from build123d import *

# Parameters (mm, degrees)
F0_W     = 4
F0_H     = 3.5
F1_DEPTH = 0.3


with BuildPart() as f1:
    # F0 (on Right) → F1 (new body)
    with BuildSketch(Plane.YZ):
        Polygon((-75.175237, 25.629358), (-80.175237, 25.629358), (-80.175237, 21.129358), (-80.175237, 20.129358), (-80.175237, 15.629358), (-75.175237, 15.629358), (-74.175237, 15.629358), (-69.175237, 15.629358), (-69.175237, 20.129358), (-69.175237, 21.129358), (-69.175237, 25.629358), (-74.175237, 25.629358), align=None)
        with Locations((-77.175237, 18.379358)):
            Rectangle(F0_W, F0_H, mode=Mode.SUBTRACT)
        with Locations((-72.175237, 18.379358)):
            Rectangle(F0_W, F0_H, mode=Mode.SUBTRACT)
        with Locations((-77.175237, 22.879358)):
            Rectangle(F0_W, F0_H, mode=Mode.SUBTRACT)
        with Locations((-72.175237, 22.879358)):
            Rectangle(F0_W, F0_H, mode=Mode.SUBTRACT)
    extrude(amount=F1_DEPTH)


solid = f1.part
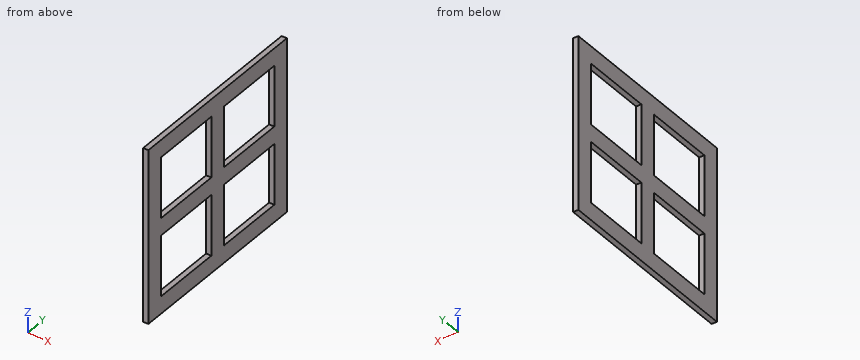
Can you work these out from the model? Positions are in its coordinate system, mm. Coordinates: 2 decimals unless noted, no trailing zeros. Loops run counter-clockwise (first coordinate to the right, second up) from the corner with the lowest first, then second, coordinate; pieces in that order, holes last. Notation, with made-up numbers: M 53.5,53 L 64.5,53 A30 ccw 64.5,80 Z; hole C -21.75,71 d4. An arc over 180 degrees is marked long. Answer as CSV lines item,"result". Start each with the question number.
1. Suppose I cut it at B-B, the plane y = -77.25. List the corners of the cut face in (x, z) for me.
2. If I drill on probe 1 along Z at (x, y) = (0.1, -76.25); probe 2 along Y at (x, z) = (0.1, 23.5), over which ranges is the centre line in solid material (lowest first)? Write a range as [from, to].
3. Suppose I cut it at C-C, the plane x = 0.2. List the corners of the cut face in (y, z) for me.
4. Suppose I cut it at A-A, the plane z = 22.25. List the corners of the cut face in (x, y) for me, plus the area to 3 significant figures.
Output:
1,outline,"M 0,15.63 L 0.3,15.63 L 0.3,16.63 L 0,16.63 Z; M 0,20.13 L 0.3,20.13 L 0.3,21.13 L 0,21.13 Z; M 0,24.63 L 0.3,24.63 L 0.3,25.63 L 0,25.63 Z"
2,probe 1,"z = [15.63, 16.63], [20.13, 21.13], [24.63, 25.63]"
2,probe 2,"y = [-80.18, -79.18], [-75.18, -74.18], [-70.18, -69.18]"
3,outline,"M -80.18,15.63 L -69.18,15.63 L -69.18,25.63 L -80.18,25.63 Z; hole M -79.18,16.63 L -75.18,16.63 L -75.18,20.13 L -79.18,20.13 Z; hole M -79.18,21.13 L -75.18,21.13 L -75.18,24.63 L -79.18,24.63 Z; hole M -74.18,16.63 L -70.18,16.63 L -70.18,20.13 L -74.18,20.13 Z; hole M -74.18,21.13 L -70.18,21.13 L -70.18,24.63 L -74.18,24.63 Z"
4,outline,"M 0,-80.18 L 0.3,-80.18 L 0.3,-79.18 L 0,-79.18 Z; M 0,-75.18 L 0.3,-75.18 L 0.3,-74.18 L 0,-74.18 Z; M 0,-70.18 L 0.3,-70.18 L 0.3,-69.18 L 0,-69.18 Z"
4,area,"0.900 mm^2"
